Design review of the part built by this model. Coordinates are the model's own, in mm. A direction names the side the tool comes from. Give positions to 0.01 mm unless a question says otherwise; leave off trailing zeros. Loops run counter-clockwise (first coordinate to the right, second up) from the corner with the lowest first, then second, coordinate; pieces in that order, holes last. Notation, with made-up numbers: (9.5, 79.5) - (49.5, 79.5) arc R38 cw to (49.5, 117.5) - close; hole circle Ø3 at (-5, -32.5). An arc over 180 degrees is marked (long way). One line per item, written item: value. Start each with the question number.
```python
from build123d import *

# Parameters (mm, degrees)
SKETCH1_W           = 50.8
SKETCH1_H           = 76.2
SKETCH1_R           = 2.4765
BOSS_EXTRUDE1_DEPTH = 6.35
SKETCH2_R           = 2.2225
BOSS_EXTRUDE2_DEPTH = 3.175
SKETCH3_W           = 6.35
SKETCH3_H           = 3.175
CUT_EXTRUDE1_DEPTH  = 10.525
SKETCH4_W           = 50.8
SKETCH4_H           = 44.45
BOSS_EXTRUDE3_DEPTH = 6.35
BOSS_EXTRUDE4_DEPTH = 22.225
SKETCH6_W           = 31.75
SKETCH6_H           = 38.1
CUT_EXTRUDE2_DEPTH  = 45.45
SKETCH7_R           = 11.1125
CUT_EXTRUDE3_DEPTH  = 7.35


with BuildPart() as part:
    # Sketch1 → Boss-Extrude1 (new body)
    with BuildSketch(Plane.XY):
        Rectangle(SKETCH1_W, SKETCH1_H)
        with Locations((-12.7, -25.4)):
            Circle(SKETCH1_R, mode=Mode.SUBTRACT)
        with Locations((12.7, -25.4)):
            Circle(SKETCH1_R, mode=Mode.SUBTRACT)
        with Locations((0, 25.4)):
            Circle(SKETCH1_R, mode=Mode.SUBTRACT)
    extrude(amount=BOSS_EXTRUDE1_DEPTH)

    # Sketch2 → Boss-Extrude2 (add)
    with BuildSketch(Plane(origin=(0, 0, 0), x_dir=(-1, 0, 0), z_dir=(0, 0, -1))):
        with Locations((-12.7, 25.4)):
            Circle(SKETCH2_R)
        with Locations((12.7, 25.4)):
            Circle(SKETCH2_R)
        with BuildLine():
            ThreePointArc((-4.7625, 13.470384182), (-7.14375, 12.373337957), (-9.2844449, 10.859638076))
            ThreePointArc((-9.2844449, 10.859638076), (-10.480991316, 10.354281134), (-11.74973534, 10.632485314))
            ThreePointArc((-11.74973534, 10.632485314), (-13.110218123, 10.843506493), (-14.257611096, 10.082630217))
            ThreePointArc((-14.257611096, 10.082630217), (-15.122968614, 8.73125), (-15.860619453, 7.306138298))
            ThreePointArc((-15.860619453, 7.306138298), (-15.94586115, 5.932028698), (-15.082870058, 4.859326635))
            ThreePointArc((-15.082870058, 4.859326635), (-14.207566158, 3.899664169), (-14.0469449, 2.610746105))
            ThreePointArc((-14.0469449, 2.610746105), (-14.2875, 0), (-14.0469449, -2.610746105))
            ThreePointArc((-14.0469449, -2.610746105), (-14.207566158, -3.899664169), (-15.082870058, -4.859326635))
            ThreePointArc((-15.082870058, -4.859326635), (-15.94586115, -5.932028698), (-15.860619453, -7.306138298))
            ThreePointArc((-15.860619453, -7.306138298), (-15.122968614, -8.73125), (-14.257611096, -10.082630217))
            ThreePointArc((-14.257611096, -10.082630217), (-13.110218123, -10.843506493), (-11.74973534, -10.632485314))
            ThreePointArc((-11.74973534, -10.632485314), (-10.480991316, -10.354281134), (-9.2844449, -10.859638076))
            ThreePointArc((-9.2844449, -10.859638076), (-7.14375, -12.373337957), (-4.7625, -13.470384182))
            ThreePointArc((-4.7625, -13.470384182), (-3.726574842, -14.253945304), (-3.333134718, -15.491811949))
            ThreePointArc((-3.333134718, -15.491811949), (-2.835643027, -16.77553519), (-1.603008357, -17.388768515))
            ThreePointArc((-1.603008357, -17.388768515), (0, -17.4625), (1.603008357, -17.388768515))
            ThreePointArc((1.603008357, -17.388768515), (2.835643027, -16.77553519), (3.333134718, -15.491811949))
            ThreePointArc((3.333134718, -15.491811949), (3.726574842, -14.253945304), (4.7625, -13.470384182))
            ThreePointArc((4.7625, -13.470384182), (7.14375, -12.373337957), (9.2844449, -10.859638076))
            ThreePointArc((9.2844449, -10.859638076), (10.480991316, -10.354281134), (11.74973534, -10.632485314))
            ThreePointArc((11.74973534, -10.632485314), (13.110218123, -10.843506493), (14.257611096, -10.082630217))
            ThreePointArc((14.257611096, -10.082630217), (15.122968614, -8.73125), (15.860619453, -7.306138298))
            ThreePointArc((15.860619453, -7.306138298), (15.94586115, -5.932028698), (15.082870058, -4.859326635))
            ThreePointArc((15.082870058, -4.859326635), (14.207566158, -3.899664169), (14.0469449, -2.610746105))
            ThreePointArc((14.0469449, -2.610746105), (14.2875, 0), (14.0469449, 2.610746105))
            ThreePointArc((14.0469449, 2.610746105), (14.207566158, 3.899664169), (15.082870058, 4.859326635))
            ThreePointArc((15.082870058, 4.859326635), (15.94586115, 5.932028698), (15.860619453, 7.306138298))
            ThreePointArc((15.860619453, 7.306138298), (15.122968614, 8.73125), (14.257611096, 10.082630217))
            ThreePointArc((14.257611096, 10.082630217), (13.110218123, 10.843506493), (11.74973534, 10.632485314))
            ThreePointArc((11.74973534, 10.632485314), (10.480991316, 10.354281134), (9.2844449, 10.859638076))
            ThreePointArc((9.2844449, 10.859638076), (7.14375, 12.373337957), (4.7625, 13.470384182))
            ThreePointArc((4.7625, 13.470384182), (3.726574842, 14.253945304), (3.333134718, 15.491811949))
            ThreePointArc((3.333134718, 15.491811949), (2.835643027, 16.77553519), (1.603008357, 17.388768515))
            ThreePointArc((1.603008357, 17.388768515), (0, 17.4625), (-1.603008357, 17.388768515))
            ThreePointArc((-1.603008357, 17.388768515), (-2.835643027, 16.77553519), (-3.333134718, 15.491811949))
            ThreePointArc((-3.333134718, 15.491811949), (-3.726574842, 14.253945304), (-4.7625, 13.470384182))
        make_face()
    extrude(amount=BOSS_EXTRUDE2_DEPTH)

    # Sketch3 → Cut-Extrude1 (cut, through all)
    with BuildSketch(Plane(origin=(0, 0, -3.175), x_dir=(-1, 0, 0), z_dir=(0, 0, -1))):
        Rectangle(SKETCH3_W, SKETCH3_H)
    extrude(amount=-CUT_EXTRUDE1_DEPTH, mode=Mode.SUBTRACT)

    # Sketch4 → Boss-Extrude3 (add)
    with BuildSketch(Plane(origin=(0, 38.1, 0), x_dir=(1, 0, 0), z_dir=(0, 1, 0))):
        with Locations((0, -28.575)):
            Rectangle(SKETCH4_W, SKETCH4_H)
    extrude(amount=-BOSS_EXTRUDE3_DEPTH)

    # Sketch5 → Boss-Extrude4 (add, symmetric)
    with BuildSketch(Plane(origin=(0, 0, 0), x_dir=(0, 0, -1), z_dir=(1, 0, 0))):
        Polygon((-44.45, 31.75), (-6.35, -6.35), (-6.35, 31.75), align=None)
    extrude(amount=BOSS_EXTRUDE4_DEPTH, both=True)

    # Sketch6 → Cut-Extrude2 (cut, through all)
    with BuildSketch(Plane.XY.offset(6.35)):
        with Locations((0, 12.7)):
            Rectangle(SKETCH6_W, SKETCH6_H)
    extrude(amount=CUT_EXTRUDE2_DEPTH, mode=Mode.SUBTRACT)

    # Sketch7 → Cut-Extrude3 (cut, through all)
    with BuildSketch(Plane.XZ.offset(-31.75)):
        with Locations((0, 25.4)):
            Circle(SKETCH7_R)
    extrude(amount=-CUT_EXTRUDE3_DEPTH, mode=Mode.SUBTRACT)


solid = part.part
```
(1) For pin 1 Ø1 at (x, y) = (18.5, 0.5) entering from -Z; pin 2 Ø8 at (x, y) = (-18.5, -22) entering from +Z; pin 3 Ø8 at (x, z) = (-8, 34.5) entering from -Y, all flat-tipped, find the tip position at first contact; note any pin that passes through.
(2) Take a section at D-D on z = 2. State the section outline as (x, y) points (1 decimal).
(3) Machinability: for faces 4 (the cylindrical face through (-3.737, 14.239, -1.565)), 5 (the cylindrical face through (-15.94, 5.91, -1.57)), 6 (the cylindrical face through (-10.499, 10.353, -1.565)), 7 (the cylindrical face through (10.499, -10.353, -1.565)), which of the approach directions +Z, -Z, +X, -X, +Y, -Y give a long, thin tool a straight path to every point of the face, cutting with its end or side? Answer none if there is none.
(4) To check wall thickness, follow L1, parallel to Y at x = 0, z = 3.25; L2, parallel to Y at x = -12.7, z = 2.25; L3, parallel to X at y = -25, z = 5. State the ranges of each line that lie inside material, in increasing order. Write a range as from..to.
(5) Draft analysis for pull direction Y (two halves, no side actions). For faces 1 (the cylindrical face through (14.2, -3.88, -1.57)), 2 (the flat face through (25.4, 14, 5)), 3 (the cylindrical face through (2.85, -16.76, -1.57)), state which applies: pulls with the +Y half, pulls with the -Y half, needs draft (parallel to the pull), parting line crosses it, or undercut.
Here are the results:
1. pin 1: z = 0
1. pin 2: z = 6.35
1. pin 3: y = 31.75
2. outline: (-25.4, -38.1) - (25.4, -38.1) - (25.4, 38.1) - (-25.4, 38.1) - close; hole circle Ø5 at (-12.7, -25.4); hole (-3.2, -1.6) - (3.2, -1.6) - (3.2, 1.6) - (-3.2, 1.6) - close; hole circle Ø5 at (0, 25.4); hole circle Ø5 at (12.7, -25.4)
3. face 4: -Z, -X, +Y
3. face 5: -Z, -X
3. face 6: -Z
3. face 7: -Z, -Y
4. L1: -38.1..-1.59, 1.59..22.92, 27.88..38.1
4. L2: -38.1..-27.88, -22.92..38.1
4. L3: -25.4..-15.14, -10.26..10.26, 15.14..25.4
5. face 1: undercut
5. face 2: needs draft
5. face 3: pulls with the -Y half
